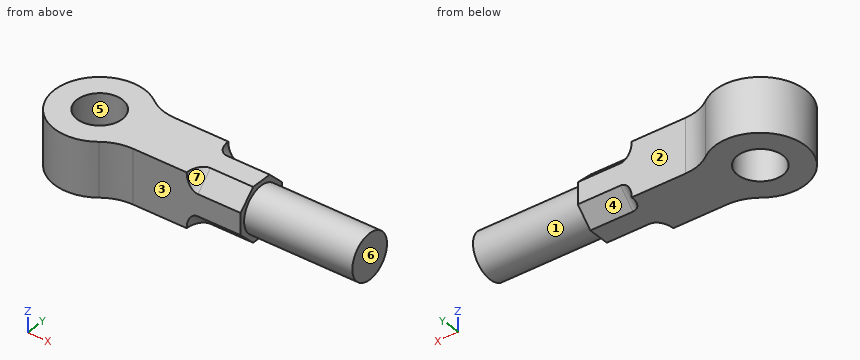
from build123d import *

# Parameters (mm, degrees)
SKETCH1_R           = 25
BOSS_EXTRUDE1_DEPTH = 30
CUT_EXTRUDE1_DEPTH  = 60
SKETCH2_3_R         = 25
BOSS_EXTRUDE2_DEPTH = 120.5
FILLET1_R           = 12.5


with BuildPart() as part:
    # Sketch1 → Boss-Extrude1 (new, symmetric)
    with BuildSketch(Plane.XY):
        with BuildLine():
            Line((60, 30), (180, 30))
            Line((180, 30), (180, -30))
            Line((180, -30), (60, -30))
            ThreePointArc((60, -30), (44.188611699, -32.565835097), (30, -40))
            ThreePointArc((30, -40), (-50, 0), (30, 40))
            ThreePointArc((30, 40), (44.188611699, 32.565835097), (60, 30))
        make_face()
        Circle(SKETCH1_R, mode=Mode.SUBTRACT)
    extrude(amount=BOSS_EXTRUDE1_DEPTH, both=True)

    # Sketch2 → Cut-Extrude1 (cut)
    with BuildSketch(Plane(origin=(180, 0, 0), x_dir=(0, 0, -1), z_dir=(1, 0, 0))):
        Polygon((-30, 11.94), (-11.94, 30), (-30, 30), align=None)
        Polygon((-30, -30), (-11.94, -30), (-30, -11.94), align=None)
        Polygon((11.94, 30), (30, 11.94), (30, 30), align=None)
        Polygon((30, -30), (30, -11.94), (11.94, -30), align=None)
    extrude(amount=-CUT_EXTRUDE1_DEPTH, mode=Mode.SUBTRACT)

    # Sketch2_3 → Boss-Extrude2 (add)
    with BuildSketch(Plane(origin=(180, 0, 0), x_dir=(0, 0, -1), z_dir=(1, 0, 0))):
        with Locations(Location((0, 0, 0), (0, 0, 90))):
            Circle(SKETCH2_3_R)
    extrude(amount=BOSS_EXTRUDE2_DEPTH)

    # Fillet1
    fillet1_edges = [part.edges().sort_by_distance(p)[0] for p in [
        (120, -20.97, 20.97),
        (120, 20.97, -20.97),
        (120, -20.97, -20.97),
        (120, 20.97, 20.97),
    ]]
    fillet(fillet1_edges, radius=FILLET1_R)


solid = part.part
Geometry: final body of the model. Coordinates: model frame, mm. Face numbers are marked on the shaded views. A direction names the side the tool comes from. Round coordinates to 2 decimals unless told otherwise and drop trailing zeros. Loops run counter-clockwise (first coordinate to the right, second up) from the corner with the lowest first, then second, coordinate; pieces in that order, holes last.
Q1. Section A-A on y = 0. Return loops of the section in (x, z), plus the area to 3 significant figures.
Q2. Access query for the marked faces 1, 2, 3 and 4. Directions: +Z, -Z, +X, -X, +Y, -Y. A direction counts if a zero-diameter tool reaches every point of the face in a straight line with its end or side. Return the directions, or none.
Q3. Material intervals for L1, parallel to Y at x = 0, z = 18.5; L2, parallel to Y at x = 103, z = 4; L3, parallel to X at y = -14, z = -21, sorted ascending.
Q4. Pull-direction query (Y, two-part tool) for the marked faces 5, 6 and 7; classes: released by +Y, released by -Y, zero draft, split by the parting line, or undercut.
Q5. Section C-C on z = 0. Return loops of the section in (x, y).
Q6. Section D-D on x = 139. Return loops of the section in (y, z).
Q7. Section B-B on x = 0. Return loops of the section in (y, z), plus the area to 3 significant figures.
Q8. Pin query (flat end, axial travel): P1, Ø1, axis at x = 130.5, z = 0, coming from the +Y side; P2, Ø8, axis at y = -9.5, z = 21.5, coming from the -X side; P3, Ø8, axis at x = 197.5, y = 14.5, coming from the +Z side. Return the tip coordinate at first contact, or that it passes through.
Evaluation:
1. outline: (-50, -30) - (-25, -30) - (-25, 30) - (-50, 30) - close; (25, -30) - (180, -30) - (180, -25) - (300.5, -25) - (300.5, 25) - (180, 25) - (180, 30) - (25, 30) - close
1. area: 16,800 mm2
2. face 1: +X
2. face 2: +Z, -Z, +X, +Y
2. face 3: +Z, -Z, +X, -Y
2. face 4: -Z, +X, +Y
3. L1: y = -50 to -25, 25 to 50
3. L2: y = -30 to 30
3. L3: x = -48 to -20.71, 20.71 to 180
4. face 5: undercut
4. face 6: zero draft
4. face 7: released by -Y
5. outline: (30, -40) arc R50 cw to (60, -30) - (180, -30) - (180, -25) - (300.5, -25) - (300.5, 25) - (180, 25) - (180, 30) - (60, 30) arc R50 cw to (30, 40) arc R50 ccw (long way) to start; hole circle Ø50 at (0, 0)
6. outline: (-30, -11.94) - (-11.94, -30) - (11.94, -30) - (30, -11.94) - (30, 11.94) - (11.94, 30) - (-11.94, 30) - (-30, 11.94) - close
7. outline: (-50, -30) - (-25, -30) - (-25, 30) - (-50, 30) - close; (25, -30) - (50, -30) - (50, 30) - (25, 30) - close
7. area: 3,000 mm2
8. P1: stops at y = 30
8. P2: stops at x = -49.7
8. P3: stops at z = 22.69
